The figure shows three views and two pictorial views of one solid part (mm, origin at its lowest corner). Answer the questions. Coordinates: 2 decimals unless noted, no trailing zeros. Write each loop counter-clockwise with the first axis right and the second up, starting at its lowest first coordinate (ties: lowest second). Pieces come first, ordered by that corner, then holes. Notation, with made-up numbers: (14, 4) - (47, 4) arc R23 ccw to (47, 34) - close; hole circle Ø5 at (-39, 60.5). An arc over 180 degrees is marked (long way). Use a Markdown table: item, result. Add a question column.
(1) The part is cut by section C-C, the plane z = 1.8. Give the vertices of the cut face in (x, y).
(2) The part is cut by section B-B, the plane x = 129.5. Give the vertices of the cut face in (y, z).
(3) The part is cut by section A-A, the plane y = 5. Give the vertices of the cut face in (x, z), then the cut area to 3 significant figures.
(4) Find the intervals of material crossed by line 1 (Y direction, x = 3.5, z = 1.5); line 2 (X direction, y = 18.75, z = 0.6), in increasing order. Write a range as from..to.
(5) Given pin 1 Ø3 at (x, y) = (3.5, 5) entering from +Z, flat-ended and moving along its own axis, determine where the tip first touches the part or whether it passes through.
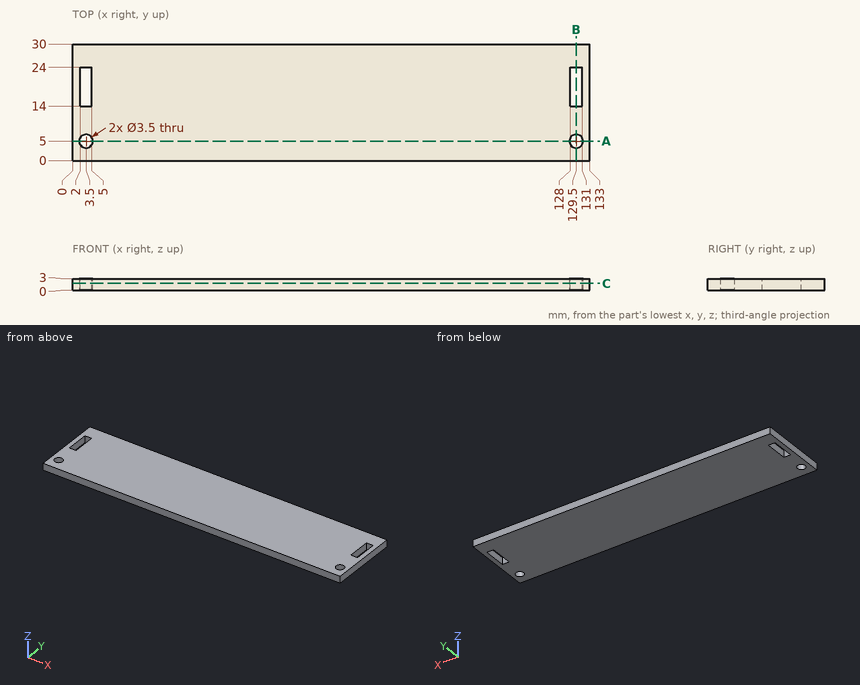
Model answer:
| question | item | result |
|---|---|---|
| 1 | outline | (0, 0) - (133, 0) - (133, 30) - (0, 30) - close; hole circle Ø3.5 at (3.5, 5); hole (2, 14) - (5, 14) - (5, 24) - (2, 24) - close; hole circle Ø3.5 at (129.5, 5); hole (128, 14) - (131, 14) - (131, 24) - (128, 24) - close |
| 2 | outline | (0, 0) - (3.25, 0) - (3.25, 3) - (0, 3) - close; (6.75, 0) - (14, 0) - (14, 3) - (6.75, 3) - close; (24, 0) - (30, 0) - (30, 3) - (24, 3) - close |
| 3 | outline | (0, 0) - (1.75, 0) - (1.75, 3) - (0, 3) - close; (5.25, 0) - (127.75, 0) - (127.75, 3) - (5.25, 3) - close; (131.25, 0) - (133, 0) - (133, 3) - (131.25, 3) - close |
| 3 | area | 378 mm^2 |
| 4 | line 1 | 0..3.25, 6.75..14, 24..30 |
| 4 | line 2 | 0..2, 5..128, 131..133 |
| 5 | pin 1 | through |
